Autodesk Inventor part; units mm, degrees
ref_plane "YZ Plane" through (0, 0, 0) normal (1, 0, 0) x (0, 1, 0)
ref_plane "XZ Plane" through (0, 0, 0) normal (0, 1, 0) x (-1, 0, 0)
ref_plane "XY Plane" through (0, 0, 0) normal (0, 0, 1) x (1, 0, 0)
sketch "Sketch1" plane through (0, 0, 0) normal (0, 0, 1) x (1, 0, 0)
  line L0 (0, 0) -> (1.8311, 0)
  line L1 (0, 0) -> (0, 45.085)
  line L2 (0.381, 45.085) -> (0.381, 0.381)
  line L3 (0.381, 0.381) -> (1.8311, 0.381)
  line L4 (1.8311, 0.381) -> (1.8311, 0)
  line L5 (0.381, 45.085) -> (0, 45.085)
  dimension "d0" = 1.8311
  dimension "d1" = 45.085
  dimension "d2" = 0.381
extrude "Extrusion1" add sketch "Sketch1" along normal blind 88.9
fillet "Fillet1" radius 2.54 2 edges at (0.1905, 45.085, 88.9) (0.1905, 45.085, 0)
sketch "Sketch2" plane through (0, 0, 0) normal (-1, 0, 0) x (0, 0, 1)
  line L0 (0, 0) -> (88.9, 0)
  circle A0 centre (40.005, 0) radius 3.175
  circle A1 centre (48.895, 0) radius 3.2307
  dimension "d6" = 6.35
  dimension "d7" = 8.89
  dimension "d8" = 40.005
extrude "Extrusion2" cut sketch "Sketch2" against normal blind 88.9
sketch "Sketch3" plane through (0, 0, 0) normal (-1, 0, 0) x (0, 0, 1)
  circle A0 centre (20.1258, 30.6113) radius 3.175
  circle A1 centre (68.8299, 30.6113) radius 3.175
  line L0 (88.9, 42.545) -> (88.9, 0)
  line L1 (0, 42.545) -> (0, 0)
  line L2 (2.54, 45.085) -> (86.36, 45.085)
  line L3 (68.8299, 30.6113) -> (48.9507, 0)
  line L4 (48.9507, 0) -> (88.9, 0)
  line L5 (20.1258, 30.6113) -> (40.005, 0)
  line L6 (0, 0.381) -> (36.8529, 0.381)
  line L7 (40.005, 0) -> (0, 0)
  point P0 (52.1257, 0)
  point P1 (36.83, 0)
  dimension "d11" = 6.35
  dimension "d12" = 6.35
  dimension "d19" = 3.175
  dimension "d20" = 3.175
  dimension "d21" = 36.4998
  dimension "d22" = 45.085
  dimension "d23" = 45.085
  dimension "d24" = 36.4998
  dimension "d25" = 57
  dimension "d26" = 57
extrude "Extrusion3" cut sketch "Sketch3" against normal blind 88.9
properties part number "Fin_full" material "Aluminum 6061"
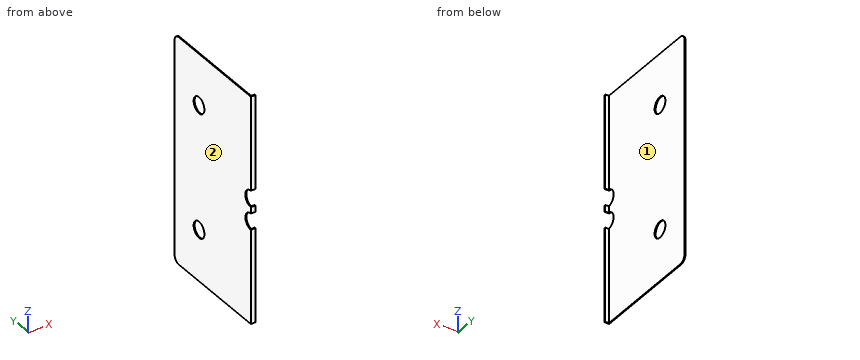
Geometry check sheet. Reference: the model listing, model coordinates, mm. Face numbers are marked on the shaded views. A direction names the side the tool comes from. Round coordinates to 2 decimals unless told otherwise and drop trailing zeros. Loops run counter-clockwise (first coordinate to the right, second up) from the corner with the lowest first, then second, coordinate; pieces in that order, holes last. Notation, with made-up numbers: (85, 8.25) - (103, 8.25) arc R15 cw to (103, 12.25) - close; hole circle Ø4 at (8.25, 89). An arc over 180 degrees is marked (long way). Write item = value, one per line. Start each with the question number.
1. Section check A-A on x = 1.35. Enter the section's corners in (y, z) (3 decimals).
2. Depth check by flat-ended pin: pin 1 (0.7 mm diameter, centred on x = 1, z = 27.5, fed in from +Y); pin 2 (1 mm diameter, centred on y = 28.5, z = 41, fed in from +X); pin 3 (2 mm diameter, centred on y = 9, z = 55.5, fed in from -X). Enter the tip coordinate at first touch or a pass-through.
3. Set-up check for the marked faces 1 and 2: record each of +Z, -Z, +X, -X, +Y, -Y from which the full face is reachable in a straight line by a thin tool's end or side.
4. Section check C-C on z = 50.5. Enter the section's corners in (x, y) (3 decimals).
5. Thickness scan on line 1 (Y direction, x = 1.4, z = 7.5); line 2 (Y direction, x = 0.2, z = 20.5) (3 decimals). Record the ranges inside material, lowest first.
6. Section check B-B on y = 7. Enter the section's corners in (x, z).
Working result:
q1.outline = (0, 0) - (0.381, 0) - (0.381, 36.853) arc R3.175 cw to (0, 36.83) - close; (0, 43.18) arc R3.175 cw to (0.381, 43.157) - (0.381, 45.687) arc R3.231 cw to (0, 45.664) - close; (0, 52.126) arc R3.231 cw to (0.381, 52.103) - (0.381, 88.9) - (0, 88.9) - close
q2.pin_1 = 0.38
q2.pin_2 = 0.38
q2.pin_3 = 0
q3.face_1 = +Z, -Z, +X, +Y
q3.face_2 = +Z, -Z, -X, +Y, -Y
q4.outline = (0, 2.804) - (0.381, 2.804) - (0.381, 45.085) - (0, 45.085) - close
q5.line_1 = 0 to 0.38
q5.line_2 = 0 to 27.458, 33.764 to 45.085
q6.outline = (0, 0) - (0.38, 0) - (0.38, 88.9) - (0, 88.9) - close
